from build123d import *

# Parameters (mm, degrees)
SKETCH1_W           = 4
SKETCH1_H           = 100
BOSS_EXTRUDE1_DEPTH = 4
SKETCH2_W           = 30
SKETCH2_H           = 50
CUT_EXTRUDE1_DEPTH  = 10


with BuildPart() as part:
    # Sketch1 → Boss-Extrude1 (new body)
    with BuildSketch(Plane(origin=(0, 0, 0), x_dir=(1, 0, 0), z_dir=(0, 1, 0))):
        Polygon((-112.5, 94), (-92.5, 94), (-92.5, 90), (-7.5, 90), (-7.5, 94), (12.5, 94), (12.5, 90), (97.5, 90), (97.5, 94), (117.5, 94), (117.5, -96), (97.5, -96), (97.5, -92), (12.5, -92), (12.5, -96), (-7.5, -96), (-7.5, -92), (-92.5, -92), (-92.5, -96), (-112.5, -96), (-112.5, -92), (-117.5, -92), (-117.5, 90), (-112.5, 90), align=None)
        with Locations((-44.11, -1)):
            Rectangle(SKETCH1_W, SKETCH1_H, mode=Mode.SUBTRACT)
    extrude(amount=BOSS_EXTRUDE1_DEPTH)

    # Sketch2 → Cut-Extrude1 (cut)
    with BuildSketch(Plane(origin=(0, 4, 0), x_dir=(1, 0, 0), z_dir=(0, 1, 0))):
        with Locations((-117.5, -1)):
            Rectangle(SKETCH2_W, SKETCH2_H)
    extrude(amount=-CUT_EXTRUDE1_DEPTH, mode=Mode.SUBTRACT)


solid = part.part
For this review, take the finished solid that the model builds, in its own axes (mm). Round coordinates to 2 decimals unless told otherwise and drop trailing zeros. Loops run counter-clockwise (first coordinate to the right, second up) from the corner with the lowest first, then second, coordinate; pieces in that order, holes last. Notation, with made-up numbers: (28.5, 51) - (64.5, 51) arc R8 ccw to (64.5, 55) - close; hole circle Ø3 at (72.5, -15). An arc over 180 degrees is marked (long way). Use one line per item in the form item = value.
1) We need section C-C on x = 22. Write out the cut boundary in (y, z).
Solutions:
outline = (0, -90) - (4, -90) - (4, 92) - (0, 92) - close
2) We need section A-A on z = -20.5. Write out the cut boundary in (x, y).
Solutions:
outline = (-102.5, 0) - (-46.11, 0) - (-46.11, 4) - (-102.5, 4) - close; (-42.11, 0) - (117.5, 0) - (117.5, 4) - (-42.11, 4) - close
3) Clearance check with flat-ended pins moving along their axes: P1, Ø2, axis at y = 2, z = -92, coming from the -X side; P2, Ø2, axis at x = -61, y = 2.5, coming from the +Z side; P3, Ø2, axis at y = 1, z = -6, coming from the -X side. State where each tip first meets the part, or that it passes through.
Solutions:
P1 = -112.5
P2 = 92
P3 = -102.5
4) Wall thickness on probe 1 along X at (y, z) = (1.1, 22.5); probe 2 along X at (y, z) = (2.3, 50); probe 3 along Z at (x, y) = (-18, 1.5): over which ranges is each line inside the solid? List them lowest first.
Solutions:
probe_1 = -102.5 to -46.11, -42.11 to 117.5
probe_2 = -117.5 to -46.11, -42.11 to 117.5
probe_3 = -90 to 92
